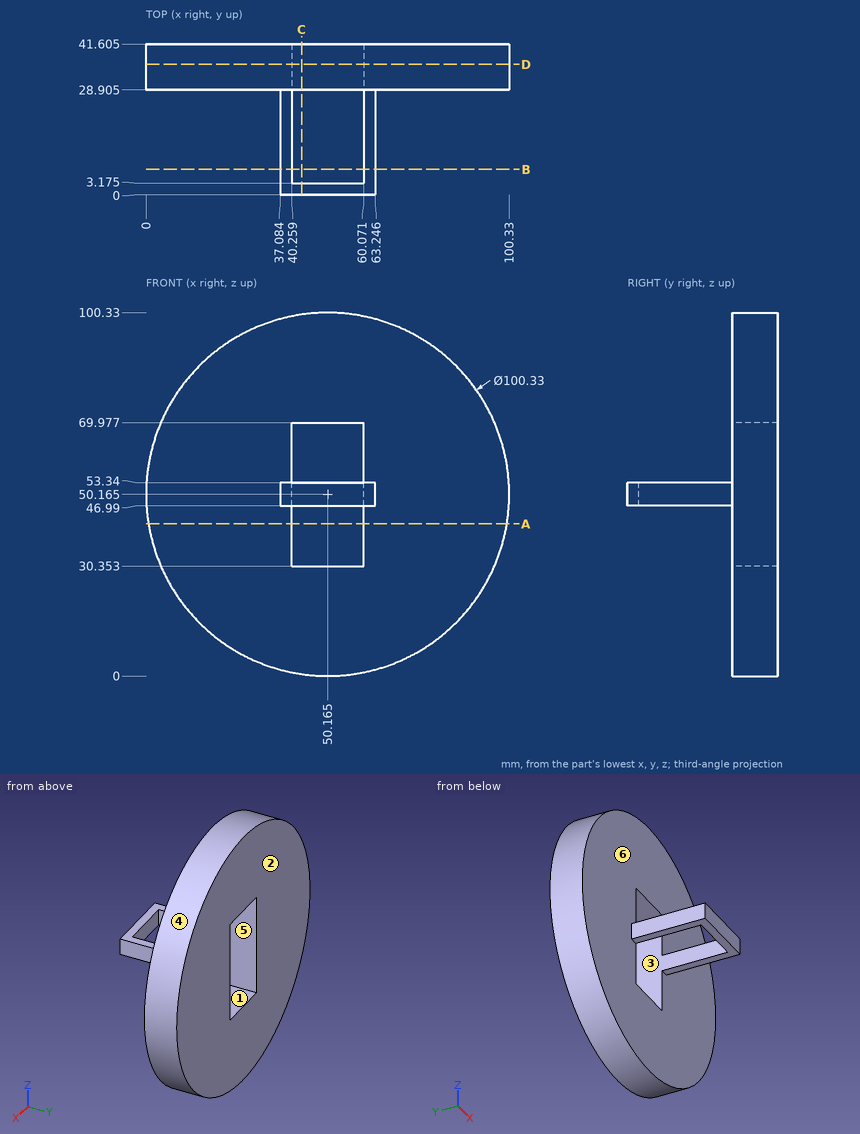
Geometry: see drawing. Coordinates: mm, zero at the bounding-box minimum. A direction names the side the tool comes from. Give positions to 0.01 mm unless a question says otherwise; leave off trailing zeros. Write each loop counter-clockwise with the first axis right and the second up, starting at its lowest first coordinate (ties: lowest second). Pieces come first, ordered by that corner, then holes. Notation, with made-up numbers: (21, -39.5) - (74, -39.5) arc R7 cw to (74, -26.5) - close; hole circle Ø4 at (-3, 29.5). An arc over 180 degrees is marked (long way). Return JSON: item names as keys, results as strings. Group by question number.
1) Mould query, pull axis Z, two halves, no side actions, for the marked faces 4, 5 and 6. Classes: released by +Z, released by -Z, zero draft, split by the parting line, or undercut.
2) Section C-C on x = 43. Return the cut outline in (y, z) (1 decimal), plus the area to 3 significant figures.
3) Section A-A on z = 42. Return the cut outline in (x, y) (1 decimal).
4) Set-up query: the marked faces 1, 2 and 3. Return all of +Z, -Z, +X, -X, +Y, -Y with unobstructed straight access to the full face (end or side cutting, diameter ignored); none if empty.
5) First-contact query: P1, Ø5, axis at x = 47.5, z = 51, coming from the +Y side (3 decimals); P2, Ø6.5, axis at x = 48, y = 35.5, coming from the +Z side; P3, Ø5, axis at x = 64, y = 6.5, coming from the +Z side; P4, Ø3, axis at x = 65, y = 6.5, coming from the -Z side. Flat tips, straight axial feed; report the tip coordinate or a pass-through.
6) Section B-B on y = 7. Return the cut outline in (x, z), plus the area to 3 significant figures.
7) Section D-D on y = 36. Return the cut outline in (x, z) (3 decimals).
8) Line query: line 1 (X direction, y = 9, z = 53); line 2 (X direction, y = 31.5, z = 51); line 3 (Y direction, x = 7, z = 68) (1 decimal). Output: solid intervals per line, ascending.
Filled in:
{
 "1": {"face 4": "split by the parting line", "face 5": "undercut", "face 6": "zero draft"},
 "2": {"outline": "(0, 47) - (3.2, 47) - (3.2, 53.3) - (0, 53.3) - close; (28.9, 0.5) - (41.6, 0.5) - (41.6, 30.4) - (28.9, 30.4) - close; (28.9, 70) - (41.6, 70) - (41.6, 99.8) - (28.9, 99.8) - close", "area": "778 mm^2"},
 "3": {"outline": "(0.7, 28.9) - (40.3, 28.9) - (40.3, 41.6) - (0.7, 41.6) - close; (60.1, 28.9) - (99.7, 28.9) - (99.7, 41.6) - (60.1, 41.6) - close"},
 "4": {"face 1": "+Y, -Y", "face 2": "+Z, -Z, +X, -X, +Y", "face 3": "+Y"},
 "5": {"P1": "stops at y = 3.175", "P2": "stops at z = 100.33", "P3": "stops at z = 53.34", "P4": "passes through"},
 "6": {"outline": "(37.08, 46.99) - (40.26, 46.99) - (40.26, 53.34) - (37.08, 53.34) - close; (60.07, 46.99) - (63.25, 46.99) - (63.25, 53.34) - (60.07, 53.34) - close", "area": "40.3 mm^2"},
 "7": {"outline": "circle Ø100.33 at (50.165, 50.165); hole (40.259, 30.353) - (60.071, 30.353) - (60.071, 69.977) - (40.259, 69.977) - close"},
 "8": {"line 1": "x = 37.08 to 40.26, 60.07 to 63.25", "line 2": "x = 0.01 to 40.26, 60.07 to 100.32", "line 3": "y = 28.9 to 41.6"}
}
